For this review, take the finished solid that the model builds, in its own axes (mm). Coordinates: 2 decimals unless noted, no trailing zeros. Write each loop counter-clockwise with the first axis right and the second up, starting at its lowest first coordinate (ties: lowest second). Pieces come first, ordered by that corner, then holes. Notation, with made-up numbers: (52.25, -27) - (82.25, -27) arc R15 cw to (82.25, -14) - close; hole circle Ø5 at (5.25, 14.25). An arc over 180 degrees is marked (long way). Use one line per item in the form item = value. Start each with the question number.
1) For L1, parallel to Z at x = -32, y = -1860; L2, parallel to Y at x = 35.5, z = 10692; L3, parallel to Y at x = 106.5, z = 10680.5, list the stretches that pass through material, from the lowest coordinate up. Write a range as from..to.
2) Insertion check: P1, Ø3, axis at x = -124.5, y = -1894.5, coming from the +Z side; P2, Ø3, axis at y = -2022.5, z = 10680.5, coming from the -X side; P3, Ø12, axis at x = 156, z = 10673, coming from the -Y side. Each pin has a flat end and moves straight along its axis. Give the tip position at first contact, or say it passes through.
3) We need section B-B (z = 10695). Give the boundary of the cut face in (x, y), plus the area to 3 significant figures.
4) We need section A-A (z = 10722). Give the boundary of the cut face in (x, y), plus the area to 3 significant figures.
Autodesk Inventor part; units mm, degrees
ref_plane "Work Plane8" through (0, -1837.3344, 10759.44) normal (0, 0, 1) x (-0.6391035, -0.7691208, 0)
ref_plane "Work Plane9" through (0, -2021.693, 10759.44) normal (0, -0.9381218, 0.3463054) x (-0.8718495, -0.1696114, -0.4594676)
ref_plane "YZ Plane" through (0, 0, 0) normal (1, 0, 0) x (0, 1, 0)
ref_plane "Work Plane8" through (0, -1837.3344, 10759.44) normal (0, 0, 1) x (-0.6391035, -0.7691208, 0)
sketch "Sketch14" plane through (0, -1837.3344, 10759.44) normal (0, 0, 1) x (-0.6391035, -0.7691208, 0)
  arc A0 (51.9231, 278.7941) -> (283.588, 0) centre (141.794, 117.8242) ccw
  arc A1 (128.7949, 130.8233) -> (154.7931, 104.8251) centre (141.794, 117.8242) ccw
  line L0 (141.794, 117.8242) -> (128.7949, 130.8233)
  line L1 (128.7949, 130.8233) -> (154.7931, 104.8251)
  point P0 (-1413.132, -1174.2468)
extrude "Extrusion9" add sketch "Sketch14" against normal blind 106.68 draft 60
ref_plane "Work Plane9" through (0, -2021.693, 10759.44) normal (0, -0.9381218, 0.3463054) x (-0.8718495, -0.1696114, -0.4594676)
sketch "Sketch15" plane through (0, -2021.693, 10759.44) normal (0, -0.9381218, 0.3463054) x (-0.8718495, -0.1696114, -0.4594676)
  line L0 (-172.5198, -77.543) -> (270.8607, -77.543)
  line L1 (270.8607, -77.543) -> (270.8607, 243.8061)
  line L2 (270.8607, 243.8061) -> (-172.5198, 243.8061)
  line L3 (-172.5198, 243.8061) -> (-172.5198, -77.543)
  point P0 (4600.712, 8189.7549)
extrude "Extrusion10" cut sketch "Sketch15" along normal blind 304.8
fillet "Fillet5" radius 60.96 1 edges at (-0.8449, -2003.3289, 10759.44)
properties part number "nose" material "Steel, Mild"
Determined:
q1.L1 = 10652.76..10674.89
q1.L2 = -2046.59..-1891.24
q1.L3 = -2050.83..-1908.92
q2.P1 = 10668.16
q2.P2 = -157.71
q2.P3 = -2055.81
q3.outline = (-127.8, -2045.48) - (127.8, -2045.48) arc R130 ccw (long way) to start
q3.area = 32,700 mm²
q4.outline = (-82.08, -2035.51) - (82.08, -2035.51) arc R83.23 ccw (long way) to start
q4.area = 13,200 mm²
